Verification items for the finished model (mm, model axes). A direction names the side the tool comes from. Give positions to 0.01 mm unless a question says otherwise; leave off trailing zeros. Write each loop counter-clockwise with the first axis right and the second up, starting at its lowest first coordinate (ties: lowest second). Pieces come first, ordered by that corner, then holes. Notation, with made-up numbers: (5.25, 9.5) - (61.25, 9.5) arc R22 ccw to (61.25, 38.5) - close; hole circle Ø10 at (29.25, -37.75). An arc over 180 degrees is marked (long way). Put each result on its own line as item: value.
from build123d import *

# Parameters (mm, degrees)
CONG_1_R = 2
CONG_2_R = 2
CONG_3_R = 0.5


with BuildPart() as part:
    # Esquisse1 → Révolution1 (revolve)
    with BuildSketch(Plane(origin=(0, 0, 0), x_dir=(0, 0, -1), z_dir=(1, 0, 0))):
        Polygon((0, 0), (15, 0), (15, 10), (3, 10), (3, 60), (1.846825454, 63.830168203), (0, 73.658150486), align=None)
    revolve(axis=Axis((0, 0, 0), (0, 1, 0)))

    # Congé1
    cong_1_edges = [part.edges().sort_by_distance(p)[0] for p in [
        (0, 10, 15),
    ]]
    fillet(cong_1_edges, radius=CONG_1_R)

    # Congé2
    cong_2_edges = [part.edges().sort_by_distance(p)[0] for p in [
        (0, 10, 3),
    ]]
    fillet(cong_2_edges, radius=CONG_2_R)

    # Congé3
    cong_3_edges = [part.edges().sort_by_distance(p)[0] for p in [
        (0, 63.830168203, 1.846825454),
    ]]
    fillet(cong_3_edges, radius=CONG_3_R)


solid = part.part
Q1. Go/stop test with flat-tipped pins: pin 1 Ø10 at (x, z) = (5, -9.5) entering from +Y; pin 2 Ø10 at (x, y) = (-4, 49.5) entering from +Z; pin 3 Ø5 at (y, z) = (59.5, 0.5) entering from +X. Record where each tip stops, or that it passes through.
Answers follow:
pin 1: stops at y = 10
pin 2: stops at z = 3
pin 3: stops at x = 3
Q2. Scan lines: line 1 along Y through (x, z) = (5.75, 3.5); line 2 along X through (y, z) = (8, 12.5); line 3 along Y through (x, z) = (13.5, -0.5). Record each from-to range of solid material in increasing order.
Answers follow:
line 1: y = 0 to 10
line 2: x = -8.29 to 8.29
line 3: y = 0 to 9.93
Q3. Section check B-B, the plane y = 11. Record the cut outline in (x, z), plus the area to 3 significant figures.
Answers follow:
outline: circle Ø6.54 at (0, 0)
area: 33.6 mm2
Q4. Section check A-A, the plane y = 39.5. Record the cut outline in (x, z).
Answers follow:
outline: circle Ø6 at (0, 0)
Q5. Set-up check for faces 1 (the face through (0, 0, 0)), 2 (the face through (0, 36, 3)): record each of +Z, -Z, +X, -X, +Y, -Y from which the full face is reachable in a straight line by a thin tool's end or side.
Answers follow:
face 1: +Z, -Z, +X, -X, -Y
face 2: +Y
